The listing builds one solid part. Answer for the finished solid, in the listing's coordinates (mm). A direction names the side the tool comes from. Give positions to 0.01 mm unless a question says otherwise; leave off trailing zeros. Write each loop counter-clockwise with the first axis right and the second up, starting at its lowest first coordinate (ties: lowest second). Pieces come first, ordered by that corner, then holes. Notation, with made-up numbers: (-10, 40) - (27, 40) arc R18 ccw to (27, 63) - close; hole circle Ø10 at (21.25, 30.25). An arc over 180 degrees is marked (long way). One line per question, with ' | ' between items. Start each with the question number.
1. A cutting plane is placed at C-C (x = 85). Determine the outline of the cut face in (y, z), then the cut area to 3 significant figures.
2. Find the intervals of material crossed by L1, parallel to Y at x = 160, z = 1.3; L2, parallel to Y at x = 12, z = 2.2; L3, parallel to X at y = 65, z = 2.35, in increasing order. Write a range as from..to.
3. The mould has two halves that part along Y. Classify faces 1 (the face through (132.089, 38.403, 1.479)), 2 (the face through (160, 69, 1)), 3 (the face through (150, 68, 1)): +Y half, -Y half, draft (parallel to the pull), parting line (faces both ways), or undercut.
4. For faces 4 (the face through (66, 20, 1)), 5 (the face through (21.265, 42.032, 1.521)), determine the directions among +Z, -Z, +X, -X, +Y, -Y from which every point of the face is accessible in a straight line to the end or side of a thin tool.
5. Given P1, Ø0.9, axis at x = 86.5, z = 1.5, coming from the +Y side; P2, Ø1.5, axis at x = 38.5, z = 2, coming from the +Y side, each flat-ended and moving along its own axis, determine where each tip first touches the part or whether it passes through.
6. A cutting plane is placed at D-D (y = 25). Determine the outline of the cut face in (x, z), then the cut area to 3 significant figures.
7. A cutting plane is placed at A-A (y = 75). Determine the outline of the cut face in (x, z).
8. A cutting plane is placed at B-B (x = 10). Determine the outline of the cut face in (y, z).
```python
from build123d import *

# Parameters (mm, degrees)
SKETCH_1_R      = 1.55
SKETCH_1_W      = 22
SKETCH_1_H      = 12
SKETCH_1_W_2    = 11
SKETCH_1_H_2    = 16
EXTRUDE_1_DEPTH = 3
FILLET_1_R      = 2


with BuildPart() as part:
    # 草图1 → 凸台-拉伸1 (new body)
    with BuildSketch(Plane.XY):
        with BuildLine():
            Line((0, 80), (0, 0))
            Line((0, 0), (170, 0))
            Line((170, 0), (170, 80))
            Line((170, 80), (150, 80))
            Line((150, 80), (150, 56.313708499))
            Line((150, 56.313708499), (113.686291501, 20))
            Line((113.686291501, 20), (94.6, 20))
            ThreePointArc((94.6, 20), (93.55, 18.95), (92.5, 20))
            Line((92.5, 20), (92.5, 23))
            Line((92.5, 23), (77.5, 23))
            Line((77.5, 23), (77.5, 20))
            ThreePointArc((77.5, 20), (76.45, 18.95), (75.4, 20))
            Line((75.4, 20), (56.313708499, 20))
            Line((56.313708499, 20), (20, 56.313708499))
            Line((20, 56.313708499), (20, 80))
            Line((20, 80), (0, 80))
        make_face()
        with Locations((10, 10)):
            Circle(SKETCH_1_R, mode=Mode.SUBTRACT)
        with Locations((25, 10)):
            Circle(SKETCH_1_R, mode=Mode.SUBTRACT)
        with Locations((42, 10)):
            Rectangle(SKETCH_1_W, SKETCH_1_H, mode=Mode.SUBTRACT)
        with Locations((69, 10)):
            Rectangle(SKETCH_1_W, SKETCH_1_H, mode=Mode.SUBTRACT)
        with Locations((10, 25)):
            Circle(SKETCH_1_R, mode=Mode.SUBTRACT)
        with Locations((10, 39)):
            Rectangle(SKETCH_1_W_2, SKETCH_1_H_2, mode=Mode.SUBTRACT)
        Polygon((45, 20), (20, 20), (20, 45), align=None, mode=Mode.SUBTRACT)
        with Locations((85, 10)):
            Circle(SKETCH_1_R, mode=Mode.SUBTRACT)
        with Locations((101, 10)):
            Rectangle(SKETCH_1_W, SKETCH_1_H, mode=Mode.SUBTRACT)
        with Locations((145, 10)):
            Circle(SKETCH_1_R, mode=Mode.SUBTRACT)
        with Locations((160, 10)):
            Circle(SKETCH_1_R, mode=Mode.SUBTRACT)
        with Locations((128, 10)):
            Rectangle(SKETCH_1_W, SKETCH_1_H, mode=Mode.SUBTRACT)
        with Locations((160, 25)):
            Circle(SKETCH_1_R, mode=Mode.SUBTRACT)
        Polygon((150, 45), (150, 20), (125, 20), align=None, mode=Mode.SUBTRACT)
        with Locations((160, 39)):
            Rectangle(SKETCH_1_W_2, SKETCH_1_H_2, mode=Mode.SUBTRACT)
        with Locations((10, 61)):
            Rectangle(SKETCH_1_W_2, SKETCH_1_H_2, mode=Mode.SUBTRACT)
        with Locations((10, 75)):
            Circle(SKETCH_1_R, mode=Mode.SUBTRACT)
        with Locations((160, 61)):
            Rectangle(SKETCH_1_W_2, SKETCH_1_H_2, mode=Mode.SUBTRACT)
        with Locations((160, 75)):
            Circle(SKETCH_1_R, mode=Mode.SUBTRACT)
    extrude(amount=EXTRUDE_1_DEPTH)

    # 圆角1
    fillet_1_edges = [part.edges().sort_by_distance(p)[0] for p in [
        (150, 20, 1.5),
        (150, 45, 1.5),
        (125, 20, 1.5),
        (20, 20, 1.5),
        (45, 20, 1.5),
        (20, 45, 1.5),
        (15.5, 31, 1.5),
        (15.5, 47, 1.5),
        (4.5, 47, 1.5),
        (4.5, 31, 1.5),
        (15.5, 53, 1.5),
        (15.5, 69, 1.5),
        (4.5, 69, 1.5),
        (4.5, 53, 1.5),
        (165.5, 31, 1.5),
        (165.5, 47, 1.5),
        (154.5, 47, 1.5),
        (154.5, 31, 1.5),
        (165.5, 53, 1.5),
        (165.5, 69, 1.5),
        (154.5, 69, 1.5),
        (154.5, 53, 1.5),
        (53, 4, 1.5),
        (53, 16, 1.5),
        (31, 16, 1.5),
        (31, 4, 1.5),
        (80, 4, 1.5),
        (80, 16, 1.5),
        (58, 16, 1.5),
        (58, 4, 1.5),
        (139, 4, 1.5),
        (139, 16, 1.5),
        (117, 16, 1.5),
        (117, 4, 1.5),
        (112, 4, 1.5),
        (112, 16, 1.5),
        (90, 16, 1.5),
        (90, 4, 1.5),
        (113.686291501, 20, 1.5),
        (150, 56.313708499, 1.5),
        (150, 80, 1.5),
        (170, 80, 1.5),
        (170, 0, 1.5),
        (0, 0, 1.5),
        (0, 80, 1.5),
        (20, 80, 1.5),
        (20, 56.313708499, 1.5),
        (56.313708499, 20, 1.5),
    ]]
    fillet(fillet_1_edges, radius=FILLET_1_R)


solid = part.part
```
Determined:
1) outline: (0, 0) - (8.45, 0) - (8.45, 3) - (0, 3) - close; (11.55, 0) - (23, 0) - (23, 3) - (11.55, 3) - close | area: 59.7 mm2
2) L1: 0..8.45, 11.55..23.45, 26.55..31, 47..53, 69..73.45, 76.55..80 | L2: 0..31, 47..53, 69..80 | L3: 0..4.5, 15.5..20, 150..154.5, 165.5..170
3) face 1: +Y half | face 2: undercut | face 3: draft
4) face 4: +Z, -Z, +Y | face 5: +Z, -Z
5) P1: y = 23 | P2: y = 38.56
6) outline: (0, 0) - (8.45, 0) - (8.45, 3) - (0, 3) - close; (11.55, 0) - (20, 0) - (20, 3) - (11.55, 3) - close; (40, 0) - (51.31, 0) - (51.31, 3) - (40, 3) - close; (118.69, 0) - (130, 0) - (130, 3) - (118.69, 3) - close; (150, 0) - (158.45, 0) - (158.45, 3) - (150, 3) - close; (161.55, 0) - (170, 0) - (170, 3) - (161.55, 3) - close | area: 169 mm2
7) outline: (0, 0) - (8.45, 0) - (8.45, 3) - (0, 3) - close; (11.55, 0) - (20, 0) - (20, 3) - (11.55, 3) - close; (150, 0) - (158.45, 0) - (158.45, 3) - (150, 3) - close; (161.55, 0) - (170, 0) - (170, 3) - (161.55, 3) - close
8) outline: (0, 0) - (8.45, 0) - (8.45, 3) - (0, 3) - close; (11.55, 0) - (23.45, 0) - (23.45, 3) - (11.55, 3) - close; (26.55, 0) - (31, 0) - (31, 3) - (26.55, 3) - close; (47, 0) - (53, 0) - (53, 3) - (47, 3) - close; (69, 0) - (73.45, 0) - (73.45, 3) - (69, 3) - close; (76.55, 0) - (80, 0) - (80, 3) - (76.55, 3) - close
